from build123d import *

# Parameters (mm, degrees)
F0_W     = 88.9
F0_H     = 88.9
F1_DEPTH = 50.8
F0_W_2   = 128.3277049661
F0_H_2   = 128.3277124166
F2_DEPTH = 25.4
F4_D     = 63.5
F6_D     = 24.892
F6_DEPTH = 63.8674141297


with BuildPart() as f1:
    # F0 (on Top) → F1 (new body)
    with BuildSketch(Plane.XY):
        with Locations((-0.7027200639, 0.5627498746)):
            Rectangle(F0_W, F0_H)
    extrude(amount=F1_DEPTH)

    # F0 (on Top) → F2 (join)
    with BuildSketch(Plane.XY):
        with Locations((-0.9680353105, 0.2974420786)):
            Rectangle(F0_W_2, F0_H_2)
        with Locations((-0.7027200639, 0.5627498746)):
            Rectangle(F0_W, F0_H, mode=Mode.SUBTRACT)
    extrude(amount=F2_DEPTH)

    # F4 (through all)
    with Locations(Plane(origin=(0, 0, 0), x_dir=(1, 0, 0), z_dir=(0, 0, -1))):
        with Locations((0, 0)):
            Hole(F4_D / 2)

    # F6 (through all, one way)
    with BuildSketch(Plane(origin=(0, 0, 0), x_dir=(1, 0, 0), z_dir=(0, 1, 0))):
        with Locations((0, -37.9534624517)):
            Circle(F6_D / 2)
    extrude(amount=-F6_DEPTH, mode=Mode.SUBTRACT)


solid = f1.part
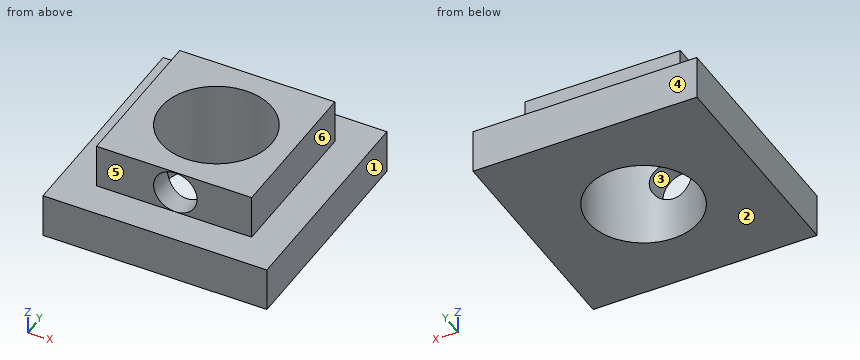
The model under review builds one solid part; all positions refer to its coordinate system, in mm. Face numbers are marked on the shaded views. A direction names the side the tool comes from. Round coordinates to 2 decimals unless told otherwise and drop trailing zeros. Loops run counter-clockwise (first coordinate to the right, second up) from the corner with the lowest first, then second, coordinate; pieces in that order, holes last. Notation, with made-up numbers: (-1, 80.25) -> (49, 80.25) arc R24 ccw to (49, 108.25) -> close; hole circle Ø9 at (53.5, 17). An arc over 180 degrees is marked (long way). Return JSON: item names as keys, results as strings.
(1) The part is to be moulded in two halves that separate along Z. For the marked faces 1, 2 and 3, say which applies: released by +Z, released by -Z, zero draft, split by the parting line, or undercut.
Solved:
{"face 1": "zero draft", "face 2": "released by -Z", "face 3": "undercut"}
(2) Add section B-B on x = 0. Write out the cut boundary in (y, z), plus the area to 3 significant figures.
Solved:
{"outline": "(-63.87, 0) -> (-31.75, 0) -> (-31.75, 25.51) -> (-43.89, 25.51) -> (-43.89, 25.4) -> (-63.87, 25.4) -> close; (-43.89, 50.4) -> (-31.75, 50.4) -> (-31.75, 50.8) -> (-43.89, 50.8) -> close; (31.75, 0) -> (64.46, 0) -> (64.46, 25.4) -> (45.01, 25.4) -> (45.01, 50.8) -> (31.75, 50.8) -> close", "area": "1,990 mm2"}
(3) Add section D-D on z = 44.5. Write out the cut boundary in (x, y).
Solved:
{"outline": "(-45.15, -43.89) -> (-10.59, -43.89) -> (-10.59, -29.93) arc R31.75 cw (long way) to (10.59, -29.93) -> (10.59, -43.89) -> (43.75, -43.89) -> (43.75, 45.01) -> (-45.15, 45.01) -> close"}
(4) For the marked faces 4, 5 and 6, list the 3-axis set-ups (+Z, -Z, +X, -X, +Y, -Y) from which the entire face can be reached by the end or side of a thin tool; tool diameter is ignored.
Solved:
{"face 4": "+Z, -Z, +X, -X, +Y", "face 5": "+Z, +X, -X, -Y", "face 6": "+Z, +X, +Y, -Y"}
(5) Add section A-A on y = 0. Write out the cut boundary in (x, z).
Solved:
{"outline": "(-65.13, 0) -> (-31.75, 0) -> (-31.75, 50.8) -> (-45.15, 50.8) -> (-45.15, 25.4) -> (-65.13, 25.4) -> close; (31.75, 0) -> (63.2, 0) -> (63.2, 25.4) -> (43.75, 25.4) -> (43.75, 50.8) -> (31.75, 50.8) -> close"}
(6) For pin 1 (20.5 mm diameter, centred on x = -3.5, z = 42.5, fed in from -Y); pin 2 (20.5 mm diameter, centred on x = 18, z = 37.5, fed in from +Y); pin 3 (5 mm diameter, centred on x = -2, z = 34, fed in from -Y), all flat-tipped, find the tip position at first contact; note any pin that passes through.
Solved:
{"pin 1": "y = -43.89", "pin 2": "y = 45.01", "pin 3": "y = 31.43"}
(7) For line 1 (Z direction, x = 0, y = -36); line 2 (Y direction, x = 0, z = 10); line 3 (X direction, y = -10.5, z = 6), list the stretches that pass through material, from the lowest coordinate up.
Solved:
{"line 1": "0 to 25.51, 50.4 to 50.8", "line 2": "-63.87 to -31.75, 31.75 to 64.46", "line 3": "-65.13 to -29.96, 29.96 to 63.2"}
(8) Add section C-C on z = 8. Write out the cut boundary in (x, y).
Solved:
{"outline": "(-65.13, -63.87) -> (63.2, -63.87) -> (63.2, 64.46) -> (-65.13, 64.46) -> close; hole circle Ø63.5 at (0, 0)"}
